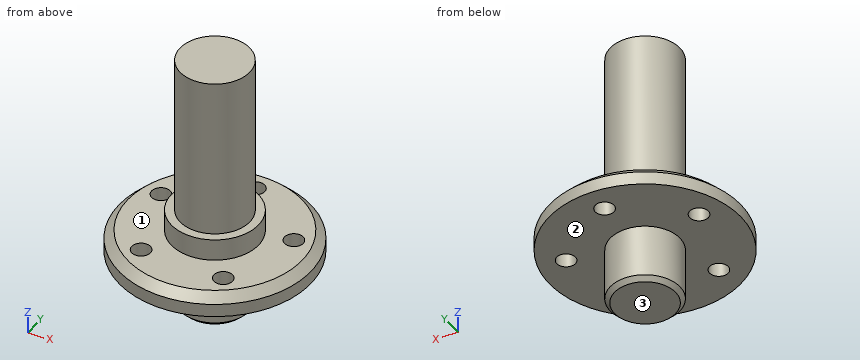
from build123d import *

# Parameters (mm, degrees)
CHAMFER1_SIZE             = 2
F_8_CLEARANCE_HOLE1_D     = 4.3053
F_8_CLEARANCE_HOLE1_DEPTH = 12
F_8_CLEARANCE_HOLE1_TIP   = 1.293442612
CHAMFER2_SIZE             = 1


with BuildPart() as part:
    # Sketch3 → Revolve1 (revolve)
    with BuildSketch(Plane(origin=(0, 0, 0), x_dir=(1, 0, 0), z_dir=(0, 1, 0))):
        Polygon((0, 0), (-8, 0), (-8, 37), (-10, 37), (-10, 42), (-22, 42), (-22, 47), (-8, 47), (-8, 60), (0, 60), align=None)
    revolve(axis=Axis((0, 0, -60), (0, 0, 1)))

    # Chamfer1
    chamfer1_edges = [part.edges().sort_by_distance(p)[0] for p in [
        (22, 0, -42),
    ]]
    chamfer(chamfer1_edges, length=CHAMFER1_SIZE)

    # #8 Clearance Hole1
    with Locations(Plane.XY.offset(-42)):
        with Locations((0, 16), (15.216904261, 4.94427191), (9.404564037, -12.94427191), (-9.404564037, -12.94427191), (-15.216904261, 4.94427191)):
            Hole(F_8_CLEARANCE_HOLE1_D / 2, depth=F_8_CLEARANCE_HOLE1_DEPTH)
            with Locations((0, 0, -(F_8_CLEARANCE_HOLE1_DEPTH + F_8_CLEARANCE_HOLE1_TIP / 2))):  # 118° drill point
                Cone(0, F_8_CLEARANCE_HOLE1_D / 2, F_8_CLEARANCE_HOLE1_TIP, mode=Mode.SUBTRACT)

    # Chamfer2
    chamfer2_edges = [part.edges().sort_by_distance(p)[0] for p in [
        (8, 0, -60),
    ]]
    chamfer(chamfer2_edges, length=CHAMFER2_SIZE)


solid = part.part
Work out the finished part from the listing and answer in its coordinate system (mm). Face numbers are marked on the shaded views. A direction names the side the tool comes from. Round coordinates to 2 decimals unless told otherwise and drop trailing zeros. Write each loop counter-clockwise with the first axis right and the second up, starting at its lowest first coordinate (ties: lowest second). Pieces come first, ordered by that corner, then holes.
1) Given pin 1 Ø5 at (x, y) = (-15.22, 4.94) entering from -Z; pin 2 Ø4 at (x, z) = (-7, -14.5) entering from -Y (3 decimals); pin 3 Ø6 at (x, y) = (11.5, -3) entering from +Z, each flat-ended and moving along its own axis, determine where each tip first touches the part or whether it passes through.
2) A cutting plane is placed at D-D (y = -12). Give the number of separate pieces and of enclosed holes in the cut face, plus the area to 3 significant figures.
3) A cutting plane is placed at C-C (z = -39). Give the vertices of the cut face in (x, y), plus the area to 3 significant figures.
4) Straight lines are drawn through the part: line 1 (Y direction, x = 0, z = -45.4); line 2 (Z direction, x = -1, y = -14.5); line 3 (Y direction, x = 0, z = -43.3). For each, find the intervals that lie inside material, in ascending order.
5) A tool of negligible diameter and unlimited length cuts with its end or side. For the marked faces 1, 2 and 3, from which of +Z, -Z, +X, -X, +Y, -Y can it reach the whole face along a straight path? Write none if from no direction.
6) A cutting plane is placed at A-A (x = 0). Give the vertices of the cut face in (y, z), plus the area to 3 significant figures.
7) A cutting plane is placed at B-B (y = 0). Give the vertices of the cut face in (x, z), plus the area to 4 significant figures.
Completed:
1. pin 1: stops at z = -47
1. pin 2: stops at y = -6.245
1. pin 3: stops at z = -37
2. separate pieces: 3
2. enclosed holes: 0
2. area: 141 mm2
3. outline: circle Ø20 at (0, 0)
3. area: 314 mm2
4. line 1: y = -22 to 13.85, 18.15 to 22
4. line 2: z = -47 to -42
4. line 3: y = -21.3 to 13.85, 18.15 to 21.3
5. face 1: +Z
5. face 2: -Z
5. face 3: -Z, +X, -X, +Y, -Y
6. outline: (-22, -47) - (-8, -47) - (-8, -59) - (-7, -60) - (7, -60) - (8, -59) - (8, -47) - (13.85, -47) - (13.85, -42) - (10, -42) - (10, -37) - (8, -37) - (8, 0) - (-8, 0) - (-8, -37) - (-10, -37) - (-10, -42) - (-20, -42) - (-22, -44) - close; (18.15, -47) - (22, -47) - (22, -44) - (20, -42) - (18.15, -42) - close
6. area: 1,090 mm2
7. outline: (-22, -47) - (-8, -47) - (-8, -59) - (-7, -60) - (7, -60) - (8, -59) - (8, -47) - (22, -47) - (22, -44) - (20, -42) - (10, -42) - (10, -37) - (8, -37) - (8, 0) - (-8, 0) - (-8, -37) - (-10, -37) - (-10, -42) - (-20, -42) - (-22, -44) - close
7. area: 1,115 mm2
